Can you work these out from the model? Positions are in its coordinate system, mm. A direction names the side the tool comes from. Coordinates: 2 decimals unless noted, no trailing zeros. Loops run counter-clockwise (first coordinate to the right, second up) from the corner with the lowest first, then second, coordinate; pieces in that order, holes last. Notation, with made-up numbers: M 17,48.25 L 46,48.25 A18 ccw 46,80.25 Z; hole C 84.5,3.5 d5. An arc over 180 degrees is marked long. Return JSON: item names as keys, results as strings. Group by question number.
```python
from build123d import *

# Parameters (mm, degrees)
SZKIC1_W                    = 31.4
SZKIC1_H                    = 17.5
DODANIE_WYCI_GNI_CIE1_DEPTH = 1.5
SZKIC2_R                    = 1.55
WYTNIJ_WYCI_GNI_CIE1_DEPTH  = 1.5
SZKIC3_W                    = 2.9
SZKIC3_H                    = 1.6
DODANIE_WYCI_GNI_CIE2_DEPTH = 1.8
SZKIC4_W                    = 3
SZKIC4_H                    = 7.5
DODANIE_WYCI_GNI_CIE3_DEPTH = 2.5
SZKIC6_W                    = 1
SZKIC6_H                    = 1
DODANIE_WYCI_GNI_CIE5_DEPTH = 5.8
SZYK_LINIOWY3_COUNT         = 3
SZYK_LINIOWY3_PITCH         = 2.5


with BuildPart() as part:
    # Szkic1 → Dodanie-wyciągnięcie1 (new body)
    with BuildSketch(Plane.XZ.offset(21.816434763)):
        with Locations((347.160462116, -460.278787137)):
            Rectangle(SZKIC1_W, SZKIC1_H)
    extrude(amount=DODANIE_WYCI_GNI_CIE1_DEPTH)

    # Szkic2 → Wytnij-wyciągnięcie1 (cut)
    with BuildSketch(Plane.XZ.offset(23.316434763)):
        with Locations((358.860462116, -465.528787137)):
            Circle(SZKIC2_R)
        with Locations((335.460462116, -455.028787137)):
            Circle(SZKIC2_R)
    extrude(amount=-WYTNIJ_WYCI_GNI_CIE1_DEPTH, mode=Mode.SUBTRACT)

    # Szkic3 → Dodanie-wyciągnięcie2 (add)
    with BuildSketch(Plane.XZ.offset(23.316434763)):
        with Locations((348.660462116, -457.028787137)):
            Rectangle(SZKIC3_W, SZKIC3_H)
    extrude(amount=DODANIE_WYCI_GNI_CIE2_DEPTH)

    # Szkic4 → Dodanie-wyciągnięcie3 (add)
    with BuildSketch(Plane.XZ.offset(23.316434763)):
        with Locations((338.960462116, -463.528787137)):
            Rectangle(SZKIC4_W, SZKIC4_H)
    extrude(amount=DODANIE_WYCI_GNI_CIE3_DEPTH)

    # Szkic6 → Dodanie-wyciągnięcie5 (add)
    with BuildSketch(Plane.ZY.offset(-337.460462116)):
        with Locations((-461.028787137, -24.566434763)):
            Rectangle(SZKIC6_W, SZKIC6_H)
    dodanie_wyci_gni_cie5 = extrude(amount=DODANIE_WYCI_GNI_CIE5_DEPTH)

    # Szyk liniowy3: Dodanie-wyciągnięcie5 ×3
    with Locations(*[(0, 0, -i * SZYK_LINIOWY3_PITCH) for i in range(1, SZYK_LINIOWY3_COUNT)]):
        add(dodanie_wyci_gni_cie5)


solid = part.part
```
1) Suppose I cut it at D-D, the plane y = -22.5. List the corners of the cut face in (x, z) for me, then the cut area to 3 significant figures.
2) For faces 1 (the face through (331.66, -24.6, -461)), 2 (the face through (334.6, -24.6, -466.529)), 3 (the face through (334.6, -24.066, -463.5)), 4 (the face through (334.6, -24.6, -465.529)), which set-ups out of +Z, -Z, +X, -X, +Y, -Y let a thin tool reach every point of the face, with its end or its side?
3) For pin 1 (0.8 mm diameter, centred on x = 338.5, y = -24.5, fed in from -Z); pin 2 (0.8 mm diameter, centred on x = 334.5, y = -24.5, fed in from -Z); pin 3 (3.5 mm diameter, centred on x = 358.86, z = -465.53, fed in from -Y), each with a flat end and sliding along its axis, tell me the tip position at first contact or that it passes through.
4) Suppose I cut it at A-A, the plane y = -24.6. List the corners of the cut face in (x, z) for me.
5) Suppose I cut it at C-C, the plane x = 358.5. List the corners of the cut face in (y, z) for me.
6) Suppose I cut it at B-B, the plane x = 339. List the corners of the cut face in (y, z) for me, then the cut area to 3 significant figures.
7) If we mould it in two halves opening along Z, with no side actions, what happens to faces 5 (the face through (349, -24, -456.229)), 6 (the face through (334.6, -24.6, -463.029)), 7 (the face through (331.46, -23, -460))? For each: +Z half, -Z half, draft (parallel to the pull), parting line (faces both ways), or undercut.
8) If I drill on line 1 (X direction, y = -22.1, z = -455); line 2 (Y direction, x = 352, z = -466.25); line 3 (X direction, y = -24, z = -457.25), over which ranges is the centre line in solid material (lowest first)? Write a range as from..to.
Returned:
{
 "1": {"outline": "M 331.46,-469.03 L 362.86,-469.03 L 362.86,-451.53 L 331.46,-451.53 Z; hole C 335.46,-455.03 d3.1; hole C 358.86,-465.53 d3.1", "area": "534 mm²"},
 "2": {"face 1": "+Z, -Z, -X, -Y", "face 2": "-Z, -X, -Y", "face 3": "+Z, -Z, -X", "face 4": "-X, -Y"},
 "3": {"pin 1": "stops at z = -467.28", "pin 2": "stops at z = -466.53", "pin 3": "stops at y = -23.32"},
 "4": {"outline": "M 331.66,-466.53 L 337.46,-466.53 L 337.46,-467.28 L 340.46,-467.28 L 340.46,-459.78 L 337.46,-459.78 L 337.46,-460.53 L 331.66,-460.53 L 331.66,-461.53 L 337.46,-461.53 L 337.46,-463.03 L 331.66,-463.03 L 331.66,-464.03 L 337.46,-464.03 L 337.46,-465.53 L 331.66,-465.53 Z; M 347.21,-457.83 L 350.11,-457.83 L 350.11,-456.23 L 347.21,-456.23 Z"},
 "5": {"outline": "M -23.32,-469.03 L -21.82,-469.03 L -21.82,-467.04 L -23.32,-467.04 Z; M -23.32,-464.02 L -21.82,-464.02 L -21.82,-451.53 L -23.32,-451.53 Z"},
 "6": {"outline": "M -25.82,-467.28 L -23.32,-467.28 L -23.32,-469.03 L -21.82,-469.03 L -21.82,-451.53 L -23.32,-451.53 L -23.32,-459.78 L -25.82,-459.78 Z", "area": "45.0 mm²"},
 "7": {"face 5": "+Z half", "face 6": "undercut", "face 7": "draft"},
 "8": {"line 1": "x = 331.46..333.91, 337.01..362.86", "line 2": "y = -23.32..-21.82", "line 3": "x = 347.21..350.11"}
}
